from build123d import *

# Parameters (mm, degrees)
BOSS_EXTRUDE1_DEPTH = 1.3
SKETCH2_W           = 11.59712349
SKETCH2_H           = 4.16940885
SKETCH2_W_2         = 9.8
SKETCH2_H_2         = 2.3
CUT_EXTRUDE1_DEPTH  = 0.1
SKETCH3_W           = 0.5
SKETCH3_H           = 0.5
CUT_EXTRUDE2_DEPTH  = 3.6


with BuildPart() as part:
    # Sketch1 → Boss-Extrude1 (new body, symmetric)
    with BuildSketch(Plane(origin=(0, 0, 0), x_dir=(1, 0, 0), z_dir=(0, 1, 0))):
        Polygon((3.75, -0.75), (6.25, -0.75), (5.75, -1.25), (4.25, -1.25), align=None)
        Polygon((8.25, -1.25), (8.75, -0.75), (6.25, -0.75), (6.75, -1.25), align=None)
        Polygon((8.75, -0.75), (6.25, -0.75), (3.75, -0.75), (3.25, -1.25), (1.75, -1.25), (1.25, -0.75), (-1.25, -0.75), (-1.25, 0.75), (-0.75, 1.25), (0.75, 1.25), (1.25, 0.75), (1.75, 1.25), (3.25, 1.25), (3.75, 0.75), (4.25, 1.25), (5.75, 1.25), (6.25, 0.75), (6.75, 1.25), (8.25, 1.25), (8.75, 0.75), align=None)
        Polygon((-1.25, -0.75), (1.25, -0.75), (0.75, -1.25), (-0.75, -1.25), align=None)
    extrude(amount=BOSS_EXTRUDE1_DEPTH, both=True)

    # Sketch2 → Cut-Extrude1 (cut)
    with BuildSketch(Plane(origin=(0, 1.3, 0), x_dir=(1, 0, 0), z_dir=(0, 1, 0))):
        with Locations((3.75, 0)):
            Rectangle(SKETCH2_W, SKETCH2_H)
        with Locations((3.75, 0)):
            Rectangle(SKETCH2_W_2, SKETCH2_H_2, mode=Mode.SUBTRACT)
    extrude(amount=-CUT_EXTRUDE1_DEPTH, mode=Mode.SUBTRACT)

    # Sketch3 → Cut-Extrude2 (cut, through all)
    with BuildSketch(Plane(origin=(0, 1.3, 0), x_dir=(1, 0, 0), z_dir=(0, 1, 0))):
        with Locations((2.5, 0)):
            Rectangle(SKETCH3_W, SKETCH3_H)
        Rectangle(SKETCH3_W, SKETCH3_H)
        with Locations((5, 0)):
            Rectangle(SKETCH3_W, SKETCH3_H)
        with Locations((7.5, 0)):
            Rectangle(SKETCH3_W, SKETCH3_H)
    extrude(amount=-CUT_EXTRUDE2_DEPTH, mode=Mode.SUBTRACT)


solid = part.part
For this review, take the finished solid that the model builds, in its own axes (mm). Give positions to 0.01 mm unless a question says otherwise; leave off trailing zeros. Order: outer loops, then holes, each group sorted by start corner. A loop starts at its lowest first (then second) coordinate and runs counter-clockwise, first axis right, second up. Notation, with made-up numbers: (61.5, 8.5) - (108.5, 8.5) arc R27 cw to (108.5, 36.5) - close; hole circle Ø3 at (-1.5, 33.25). An arc over 180 degrees is marked (long way). Answer as a JSON object with one key per item and string values. Group by question number.
Item 1: Take a section at D-D on x = 1.5. Give the boundary of the cut face in (y, z).
Item 2: Take a section at B-B on z = -0.1. Give the boundary of the cut face in (x, y).
Item 3: Take a section at A-A on x = 0. Give the boundary of the cut face in (y, z).
Item 4: Wall thickness on line 1 along X through (y, z) = (-0.65, -0.2); line 2 along X through (y, z) = (0.05, 1.1); line 3 along X through (y, z) = (-0.05, 1): over which ranges is each line inside the solid? List them lowest first.
Item 5: Take a section at C-C on y = 0.5. Give the number of separate pieces and of enclosed holes in the cut face, and give its area (3 significant figures).
Reported:
{
 "1": {"outline": "(-1.3, -1) - (1.3, -1) - (1.3, 1) - (-1.3, 1) - close"},
 "2": {"outline": "(-1.25, -1.3) - (-0.25, -1.3) - (-0.25, 1.3) - (-1.15, 1.3) - (-1.15, 1.2) - (-1.25, 1.2) - close; (0.25, -1.3) - (2.25, -1.3) - (2.25, 1.3) - (0.25, 1.3) - close; (2.75, -1.3) - (4.75, -1.3) - (4.75, 1.3) - (2.75, 1.3) - close; (5.25, -1.3) - (7.25, -1.3) - (7.25, 1.3) - (5.25, 1.3) - close; (7.75, -1.3) - (8.75, -1.3) - (8.75, 1.2) - (8.65, 1.2) - (8.65, 1.3) - (7.75, 1.3) - close"},
 "3": {"outline": "(-1.3, -1.25) - (1.2, -1.25) - (1.2, -1.15) - (1.3, -1.15) - (1.3, -0.25) - (-1.3, -0.25) - close; (-1.3, 0.25) - (1.3, 0.25) - (1.3, 1.15) - (1.2, 1.15) - (1.2, 1.25) - (-1.3, 1.25) - close"},
 "4": {"line 1": "-1.25 to -0.25, 0.25 to 2.25, 2.75 to 4.75, 5.25 to 7.25, 7.75 to 8.75", "line 2": "-0.9 to 0.9, 1.6 to 3.4, 4.1 to 5.9, 6.6 to 8.4", "line 3": "-1 to 1, 1.5 to 3.5, 4 to 6, 6.5 to 8.5"},
 "5": {"separate pieces": "1", "enclosed holes": "4", "area": "22.0 mm^2"}
}
